Autodesk Inventor part; units mm, degrees
ref_plane "YZ Plane" through (0, 0, 0) normal (1, 0, 0) x (0, 1, 0)
ref_plane "XZ Plane" through (0, 0, 0) normal (0, 1, 0) x (-1, 0, 0)
ref_plane "XY Plane" through (0, 0, 0) normal (0, 0, 1) x (1, 0, 0)
sketch "Sketch1" plane through (0, 0, 0) normal (0, 1, 0) x (-1, 0, 0)
  line L0 (28.75, 9.525) -> (-28.75, 9.525) construction
  line L1 (-28.75, 9.525) -> (-28.75, -9.525) construction
  line L2 (-28.75, -9.525) -> (28.75, -9.525) construction
  line L3 (28.75, -9.525) -> (28.75, 9.525) construction
  line L4 (28.75, 9.525) -> (-28.75, -9.525) construction
  line L5 (-28.75, 9.525) -> (28.75, -9.525) construction
  circle A0 centre (28.75, 9.525) radius 2.65
  circle A1 centre (28.75, -9.525) radius 2.65
  circle A2 centre (-28.75, 9.525) radius 2.65
  circle A3 centre (-28.75, -9.525) radius 2.65
  line L6 (36.4, 17.175) -> (-36.4, 17.175)
  line L7 (-36.4, 17.175) -> (-36.4, -17.175)
  line L8 (-36.4, -17.175) -> (36.4, -17.175)
  line L9 (36.4, -17.175) -> (36.4, 17.175)
  line L10 (36.4, 17.175) -> (-36.4, -17.175) construction
  line L11 (-36.4, 17.175) -> (36.4, -17.175) construction
  point P0 (0, 0)
  dimension "d0" = 19.05
  dimension "d1" = 57.5
  dimension "d2" = 5.3
  dimension "d3" = 5
  dimension "d4" = 5
extrude "Extrusion1" add sketch "Sketch1" along normal blind 3
sketch "Sketch2" plane through (0, 3, 0) normal (0, 1, 0) x (1, 0, 0)
  line L0 (36.4, -17.175) -> (36.4, 17.175)
  line L1 (36.4, 17.175) -> (-36.4, 17.175)
  line L2 (-36.4, 17.175) -> (-36.4, -17.175)
  line L3 (-36.4, -17.175) -> (36.4, -17.175)
  circle A0 centre (-28.75, -9.525) radius 2.65
  circle A1 centre (-28.75, 9.525) radius 2.65
  circle A2 centre (28.75, -9.525) radius 2.65
  circle A3 centre (28.75, 9.525) radius 2.65
  line L4 (-24.375, 17.175) -> (-33.125, 17.175)
  line L5 (-33.125, 17.175) -> (-33.125, -17.175)
  line L6 (-33.125, -17.175) -> (-24.375, -17.175)
  line L7 (-24.375, -17.175) -> (-24.375, 17.175)
  line L8 (-28.75, -17.175) -> (-28.75, 17.175) construction
  line L9 (33.125, 17.175) -> (24.375, 17.175)
  line L10 (24.375, 17.175) -> (24.375, -17.175)
  line L11 (24.375, -17.175) -> (33.125, -17.175)
  line L12 (33.125, -17.175) -> (33.125, 17.175)
  line L13 (28.75, 17.175) -> (28.75, -17.175) construction
  line L14 (36.4, 17.175) -> (-36.4, 17.175)
  line L15 (-36.4, -17.175) -> (36.4, -17.175)
  dimension "d14" = 8.75
extrude "Extrusion2" add sketch "Sketch2" along normal blind 1.35 contours L3 L10 L1 L12 | L3 L5 L1 L7
chamfer "Chamfer2" distance 1.35 angle 45 4 edges at (-33.125, 4.35, 0) (-24.375, 4.35, 0) (24.375, 4.35, 0) (33.125, 4.35, 0)
properties part number "Platina" material "PET Plastic"
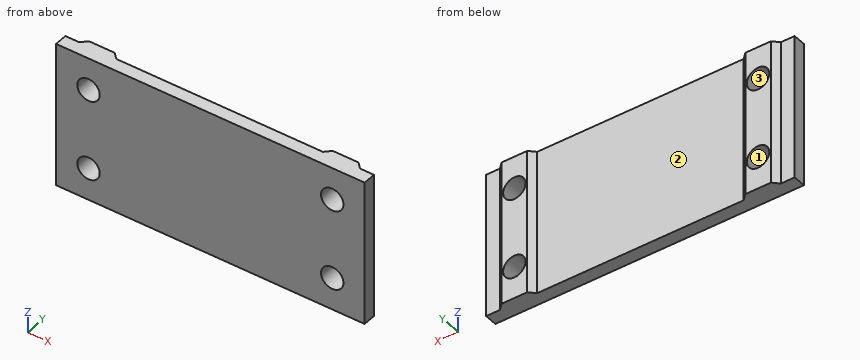
The listing builds one solid part. Answer for the finished solid, in the listing's coordinates (mm). Face numbers are marked on the shaded views. Round coordinates to 2 decimals unless told otherwise and drop trailing zeros. Write each loop counter-clockwise with the first axis right and the second up, starting at its lowest first coordinate (ties: lowest second). Pieces come first, ordered by that corner, then holes. Notation, with made-up numbers: (80, -30.5) - (106, -30.5) arc R22 cw to (106, -6.5) - close; hole circle Ø1 at (89.25, 30.25). An arc over 180 degrees is marked (long way). Use a Markdown table: item, result. Add a question column.
1. The part is cut by section D-D (x = -20). Write down the section's boundary in (y, z) (3 decimals), and give its area (3 significant figures).
2. Consider line 1 (Z direction, x = 28.75, y = 1.5) (3 decimals); line 2 (X direction, y = 1, z = -8); line 3 (X direction, y = 0.6, z = -11.5). Determine where each line is inside the solid, lowest interval first.
3. The part is cut by section C-C (y = 1.85). Write down the section's boundary in (x, z) (3 decimals).
4. For a pull along Z with two mould halves and no side action, classify the marked faces 1, 2 and 3 as +Z half, -Z half, draft (parallel to the pull), parting line (faces both ways), or undercut.
5. Flat-ended cylindrical pins translate along their axes: P1, Ø2.5, axis at x = 35, z = -7.5, coming from the +Y side; P2, Ø3.5, axis at x = -34, z = -1, coming from the +Y side. Find the tip coordinate at first contact, or state that the pin passes through.
Reported:
| question | item | result |
|---|---|---|
| 1 | outline | (0, -17.175) - (3, -17.175) - (3, 17.175) - (0, 17.175) - close |
| 1 | area | 103 mm^2 |
| 2 | line 1 | -17.175 to -12.175, -6.875 to 6.875, 12.175 to 17.175 |
| 2 | line 2 | -36.4 to -30.92, -26.58 to 26.58, 30.92 to 36.4 |
| 2 | line 3 | -36.4 to -30.52, -26.98 to 26.98, 30.52 to 36.4 |
| 3 | outline | (-36.4, -17.175) - (36.4, -17.175) - (36.4, 17.175) - (-36.4, 17.175) - close; hole circle Ø5.3 at (-28.75, -9.525); hole circle Ø5.3 at (-28.75, 9.525); hole circle Ø5.3 at (28.75, -9.525); hole circle Ø5.3 at (28.75, 9.525) |
| 4 | face 1 | undercut |
| 4 | face 2 | draft |
| 4 | face 3 | undercut |
| 5 | P1 | y = 3 |
| 5 | P2 | y = 3.88 |
